from build123d import *

# Parameters (mm, degrees)
F0_R          = 5.5
F1_DEPTH      = 60
F4_DEPTH      = 26
F4_DEPTH_BACK = 26
F5_R          = 4
F6_DEPTH      = 5
F7_R          = 4
F8_DEPTH      = 15
F9_R          = 11
F10_DEPTH     = 10.001
F11_R         = 6
F12_DEPTH     = 25


# Not quite as in the source:
# - a feature names something its author has since deleted; it is built from what else it names


with BuildPart() as f1:
    # F0 (on Front) → F1 (new body)
    with BuildSketch(Plane.XZ):
        with BuildLine():
            ThreePointArc((-0.0872969156, -53.4805140133), (-11.9999962709, -41.4659778258), (-0.0575900904, -29.4809696761))
            Line((-0.0575900904, -29.4809696761), (-5.4639e-06, 17.0404876904))
            Line((-5.4639e-06, 17.0404876904), (-70.0428405992, 17.0404876904))
            Line((-70.0428405992, 17.0404876904), (-70.0428405992, 7.0404876904))
            Line((-70.0428405992, 7.0404876904), (-20.0428405992, 7.0404876904))
            Line((-20.0428405992, 7.0404876904), (-20.6929361639, -127.9595123096))
            Line((-20.6929361639, -127.9595123096), (-70.6929361639, -127.9595123096))
            Line((-70.6929361639, -127.9595123096), (-70.6929361639, -137.9595123096))
            Line((-70.6929361639, -137.9595123096), (-0.1918656855, -137.9595123096))
            Line((-0.1918656855, -137.9595123096), (-0.1862936956, -133.4580141387))
            ThreePointArc((-0.1862936956, -133.4580141387), (-11.9988136294, -121.4446249335), (-0.1565894029, -109.4605157571))
            Line((-0.1565894029, -109.4605157571), (-0.0872969156, -53.4805140133))
        make_face()
        with Locations((-9.947382845, -81.480831509)):
            Circle(F0_R, mode=Mode.SUBTRACT)
    extrude(amount=F1_DEPTH)


with BuildPart() as f1_1:
    # F2: moved
    add(f1.part.moved(Location((0, 30, 0))))

    # F3 (on Front) → F4 (cut, two sides)
    with BuildSketch(Plane.XZ) as f4_sk:
        with BuildLine():
            ThreePointArc((0, -55.5154254436), (-14, -41.5154254436), (0, -27.5154254436))
            Line((0, -27.5154254436), (0, -26.5154254436))
            ThreePointArc((0, -26.5154254436), (-15, -41.5154254436), (0, -56.5154254436))
            Line((0, -56.5154254436), (0, -55.5154254436))
        make_face()
        with BuildLine():
            Line((0, -107.5154236555), (0, -106.5154236555))
            ThreePointArc((0, -106.5154236555), (-15, -121.5154236555), (0, -136.5154236555))
            Line((0, -136.5154236555), (0, -135.5154236555))
            ThreePointArc((0, -135.5154236555), (-14, -121.5154236555), (0, -107.5154236555))
        make_face()
    extrude(amount=F4_DEPTH, mode=Mode.SUBTRACT)
    extrude(f4_sk.sketch, amount=-F4_DEPTH_BACK, mode=Mode.SUBTRACT)

    # F5 (on face) → F6 (cut)
    with BuildSketch(Plane.XY.offset(-127.9595123096)):
        with Locations((-40.0428405992, -20)):
            Circle(F5_R)
        with Locations((-40.0428405992, 20)):
            Circle(F5_R)
    extrude(amount=-F6_DEPTH, mode=Mode.SUBTRACT)

    # F7 (on face) → F8 (cut)
    with BuildSketch(Plane.XY.offset(17.0404876904)):
        with Locations((-40.0428405992, 20)):
            Circle(F7_R)
        with Locations((-40.2286797762, -20)):
            Circle(F7_R)
    extrude(amount=-F8_DEPTH, mode=Mode.SUBTRACT)

    # F9 (on face) → F10 (cut, through all)
    with BuildSketch(Plane.XY.offset(-127.9595123096)):
        with Locations((-40.0215312839, 0)):
            Circle(F9_R)
    extrude(amount=-F10_DEPTH, mode=Mode.SUBTRACT)

    # F11 (on face) → F12 (cut)
    with BuildSketch(Plane.XY.offset(17.0404876904)):
        with Locations((-40.0154478848, 0)):
            Circle(F11_R)
    extrude(amount=-F12_DEPTH, mode=Mode.SUBTRACT)


solid = f1_1.part
Verification items for the finished model (mm, model axes). A direction names the side the tool comes from. Give positions to 0.01 mm unless a question says otherwise; leave off trailing zeros. Write each loop counter-clockwise with the first axis right and the second up, starting at its lowest first coordinate (ties: lowest second). Pieces come first, ordered by that corner, then holes.
(1) Cross-section at B-B (x = -60). Enter the section's corners in (y, z), plus the area to 3 significant figures.
(2) Mould release check, pull along Y, two halves, no side actions. Record for faces 6 (the face through (-20, -30, -59)), 7 (the face through (-20, 30, -59)), 8 (the face through (-12, 0.4, -41.7)), 9 (the face through (-13.997, 0.364, -41.805)): +Y half, -Y half, draft (parallel to the pull), parting line (faces both ways), or undercut.
(3) Cross-section at A-A (x = -10). State how many separate pieces and enclosed holes the cut face has, plus the area to 3 significant figures.
(4) Material ranges on line 1 (Z direction, x = -47, y = 11); line 2 (Z direction, x = -29.5, y = 1); line 3 (X direction, y = -11.5, z = -120.5), recorded low to high.
(5) Gauge pin test, flat ends, axial feed: pin 1 (5 mm diameter, centred on y = -13, z = 12, fed in from -X); pin 2 (5 mm diameter, centred on y = 19, z = -34, fed in from -X); pin 3 (6.5 mm diameter, centred on x = -40, y = -20, fed in from +Z). Record the tip position at first contact, or that the pin passes through.
(6) Cross-section at C-C (y = 14). Enter the section's corners in (x, z).
(7) Cross-section at D-D (z = -77.5). Enter the section's corners in (x, y), plus the area to 3 significant figures.
(8) Access from +Z, -Z, +X, -X, +Y, -Y to the whole of each face (thin tool, end or side, straight path). Record for faces 1 (the face through (-51, 7, -127.96)), 2 (the face through (-36.228, 21.201, -130.425)), 3 (the face through (-35, 7, 17.04)), 4 (the face through (-13.997, -0.364, -121.804)), 5 (the face through (-70.043, 0, 12)).
Worked out:
1. outline: (-30, -137.96) - (30, -137.96) - (30, -127.96) - (-30, -127.96) - close; (-30, 7.04) - (30, 7.04) - (30, 17.04) - (-30, 17.04) - close
1. area: 1,200 mm2
2. face 6: -Y half
2. face 7: +Y half
2. face 8: draft
2. face 9: undercut
3. separate pieces: 4
3. enclosed holes: 4
3. area: 6,760 mm2
4. line 1: z = -137.96 to -127.96, 7.04 to 17.04
4. line 2: z = 7.04 to 17.04
4. line 3: x = -20.66 to -14.97, -13.96 to -11.96
5. pin 1: stops at x = -70.04
5. pin 2: stops at x = -20.25
5. pin 3: stops at z = -132.96
6. outline: (-70.69, -137.96) - (-0.19, -137.96) - (-0.19, -136.51) arc R15 cw to (-0.15, -106.52) - (-0.09, -56.52) arc R15 cw to (-0.05, -26.52) - (0, 17.04) - (-70.04, 17.04) - (-70.04, 7.04) - (-20.04, 7.04) - (-20.69, -127.96) - (-70.69, -127.96) - close; (-0.19, -135.51) - (-0.19, -133.46) arc R12 cw to (-0.16, -109.46) - (-0.15, -107.52) arc R14 ccw to start; (-0.09, -55.52) - (-0.09, -53.48) arc R12 cw to (-0.06, -29.48) - (-0.06, -27.52) arc R14 ccw to start; hole circle Ø11 at (-9.95, -81.48)
7. outline: (-20.45, -30) - (-13.74, -30) - (-13.74, 30) - (-20.45, 30) - close; (-6.15, -30) - (-0.12, -30) - (-0.12, 30) - (-6.15, 30) - close
7. area: 765 mm2
8. face 1: -X, +Y, -Y
8. face 2: +Z
8. face 3: +Z, +X, -X, +Y, -Y
8. face 4: none
8. face 5: +Z, -X, +Y, -Y
